Autodesk Inventor part; units mm, degrees
ref_plane "YZ Plane" through (0, 0, 0) normal (1, 0, 0) x (0, 1, 0)
ref_plane "XZ Plane" through (0, 0, 0) normal (0, 1, 0) x (-1, 0, 0)
ref_plane "XY Plane" through (0, 0, 0) normal (0, 0, 1) x (1, 0, 0)
sketch "Sketch1" plane through (0, 0, 0) normal (0, 1, 0) x (-1, 0, 0)
  line L0 (39.28, 27.305) -> (-39.28, 27.305)
  line L1 (-39.28, 27.305) -> (-39.28, -27.305)
  line L2 (-39.28, -27.305) -> (39.28, -27.305)
  line L3 (39.28, -27.305) -> (39.28, 27.305)
  line L4 (39.28, 27.305) -> (-39.28, -27.305) construction
  line L5 (-39.28, 27.305) -> (39.28, -27.305) construction
  circle A0 centre (-34.28, 0) radius 1.75
  circle A1 centre (34.28, 0) radius 1.75
  line L6 (29.28, -5) -> (2.28, -5)
  line L7 (2.28, -5) -> (2.28, 5)
  line L8 (2.28, 5) -> (29.28, 5)
  line L9 (29.28, 5) -> (29.28, -5)
  line L10 (29.28, -5) -> (2.28, 5) construction
  line L11 (2.28, -5) -> (29.28, 5) construction
  line L12 (-29.28, 5) -> (-2.28, 5)
  line L13 (-2.28, 5) -> (-2.28, -5)
  line L14 (-2.28, -5) -> (-29.28, -5)
  line L15 (-29.28, -5) -> (-29.28, 5)
  line L16 (-29.28, 5) -> (-2.28, -5) construction
  line L17 (-2.28, 5) -> (-29.28, -5) construction
  point P0 (0, 0)
  point P1 (15.78, 0)
  point P2 (-15.78, 0)
  dimension "d0" = 78.56
  dimension "d1" = 54.61
  dimension "d2" = 3.5
  dimension "d3" = 5
  dimension "d4" = 3.5
  dimension "d5" = 5
  dimension "d6" = 27
  dimension "d7" = 10
  dimension "d8" = 5
  dimension "d9" = 27
  dimension "d10" = 10
  dimension "d11" = 5
  dimension "d16" = 68.56
extrude "Extrusion1" add sketch "Sketch1" along normal blind 1.7
extrude "Extrusion2" add sketch "Sketch1" along normal blind 16.58 contours L6 L7 L8 L9 | L12 L13 L14 L15
sketch "Sketch2" plane through (0, 1.7, 0) normal (0, 1, 0) x (1, 0, 0)
  line L0 (-13.9986, -11.26) -> (17.2433, -11.26) construction
  line L1 (17.2433, -11.26) -> (17.2433, -14.9075) construction
  line L2 (17.2433, -14.9075) -> (-13.9986, -14.9075) construction
  line L3 (-13.9986, -14.9075) -> (-13.9986, -11.26) construction
  point P0 (0, 0)
properties part number "powerdiset"
Here's how the part is built. I have some questions about the finished solid (model axes, mm). A direction names the side the tool comes from. Give positions to 0.01 mm unless a question says otherwise; leave off trailing zeros. Loops run counter-clockwise (first coordinate to the right, second up) from the corner with the lowest first, then second, coordinate; pieces in that order, holes last. Notation, with made-up numbers: (-26.75, 84) -> (31.25, 84) arc R19 ccw to (31.25, 99) -> close; hole circle Ø9 at (-30.5, 28.25). An arc over 180 degrees is marked (long way). One line per item, written item: value.
Q1. We'd pull the mould along Z, two halves only. Please class faces 1 (the face through (-35.897, 0.838, 0.67)), 2 (the face through (-1, 1, 27.305)), 3 (the face through (1, 0, 0)), 4 (the face through (36.03, 0.84, -0.08)): pulls with the +Z half, pulls with the -Z half, needs draft (parallel to the pull), parting line crosses it, or undercut.
Answers follow:
face 1: undercut
face 2: pulls with the +Z half
face 3: needs draft
face 4: undercut
Q2. Suppose I cut it at D-D on x = -22. Please give me the cut outline in (y, z) (3 decimals), then the cut area to 3 significant figures.
Answers follow:
outline: (0, -27.305) -> (1.7, -27.305) -> (1.7, -5) -> (16.58, -5) -> (16.58, 5) -> (1.7, 5) -> (1.7, 27.305) -> (0, 27.305) -> close
area: 242 mm^2
Q3. Suppose I cut it at B-B on x = -34.28. Please give me the cut outline in (y, z) (3 decimals), then the cut area to 3 significant figures.
Answers follow:
outline: (0, -27.305) -> (1.7, -27.305) -> (1.7, -1.75) -> (0, -1.75) -> close; (0, 1.75) -> (1.7, 1.75) -> (1.7, 27.305) -> (0, 27.305) -> close
area: 86.9 mm^2
Q4. Suppose I cut it at A-A on y = 5.75. Please give me the cut outline in (x, z), then the cut area to 3 significant figures.
Answers follow:
outline: (-29.28, -5) -> (-2.28, -5) -> (-2.28, 5) -> (-29.28, 5) -> close; (2.28, -5) -> (29.28, -5) -> (29.28, 5) -> (2.28, 5) -> close
area: 540 mm^2
Q5. On a 3-axis mill with a long thin cutter (end or side, diameter ignored), from which of +Z, -Z, +X, -X, +Y, -Y can I reach the whole of each face in a straight line? I mean faces 5 (the face through (2.28, 9, 0)), 6 (the face through (29.28, 9, 0)), 7 (the face through (16, 9, -5)), 8 (the face through (16, 9, 5)). Say none if no direction works.
Answers follow:
face 5: +Z, -Z, +Y
face 6: +Z, -Z, +X, +Y
face 7: -Z, +X, -X, +Y
face 8: +Z, +X, -X, +Y
Q6. If I drill on line 1 along Z through (x, y) = (34.28, 0.9) (3 decimals); line 2 along Y through (x, z) = (-1.5, -15.5); line 3 along X through (y, z) = (14, -4.5), over which ranges is the centre line in solid material (lowest first)?
Answers follow:
line 1: -27.305 to -1.75, 1.75 to 27.305
line 2: 0 to 1.7
line 3: -29.28 to -2.28, 2.28 to 29.28
Q7. Suppose I cut it at C-C on z = 0. Please give me the cut outline in (x, y).
Answers follow:
outline: (-39.28, 0) -> (-36.03, 0) -> (-36.03, 1.7) -> (-39.28, 1.7) -> close; (-32.53, 0) -> (32.53, 0) -> (32.53, 1.7) -> (29.28, 1.7) -> (29.28, 16.58) -> (2.28, 16.58) -> (2.28, 1.7) -> (-2.28, 1.7) -> (-2.28, 16.58) -> (-29.28, 16.58) -> (-29.28, 1.7) -> (-32.53, 1.7) -> close; (36.03, 0) -> (39.28, 0) -> (39.28, 1.7) -> (36.03, 1.7) -> close
Q8. I'm going to push flat-ended pins straight in: pin 1 Ø10 at (x, z) = (-24.5, 21) entering from -Y; pin 2 Ø5.5 at (x, z) = (-34.28, 0) entering from +Y; pin 3 Ø1.5 at (y, z) = (8.5, 2.5) entering from -X; pin 4 Ø7.5 at (x, y) = (-14, 8.5) entering from -Z. Where does each tip first touch, or does it pass through?
Answers follow:
pin 1: y = 0
pin 2: y = 1.7
pin 3: x = -29.28
pin 4: z = -5
